Verification items for the finished model (mm, model axes). Face numbers are marked on the shaded views. A direction names the side the tool comes from. Give positions to 0.01 mm unless a question says otherwise; leave off trailing zeros. Order: outer loops, then holes, each group sorted by start corner. A loop starts at its lowest first (then second) coordinate and runs counter-clockwise, first axis right, second up. Notation, with made-up numbers: (81.5, -8.5) -> (86.5, -8.5) arc R28 cw to (86.5, 14.5) -> close; hole circle Ø9 at (7, -24). An arc over 180 degrees is marked (long way). Return JSON: item names as keys, results as strings. Group by question number.
(1) Tool access check on the marked faces 1 and 2. Record the directions out of +Z, -Z, +X, -X, +Y, -Y that give a thin tool (end or side, any length) a straight path to the whole face; none if there is none.
(2) Cross-section at A-A on y = 0. Enter the section's corners in (x, z).
(3) Thickness scan on line 1 along Z through (x, y) = (9.75, 0.25); line 2 along Y through (x, z) = (1.25, 3.5); line 3 along Y through (x, z) = (4.75, 4.75). Record the ranges inside material, lowest first.
(4) Depth check by flat-ended pin: pin 1 Ø3 at (x, z) = (4.5, 9) entering from +Y; pin 2 Ø1 at (y, z) = (7.5, 13) entering from +X; pin 3 Ø1.5 at (y, z) = (10, 9) entering from +X. Enter the tip coordinate at first touch or a pass-through.
(5) Cross-section at B-B on z = 13.5. Enter the section's corners in (x, y).
(6) Release check for a two-part mould opening along Y. For the marked faces 3, 4 and 5 record: pulls with the +Y half, pulls with the -Y half, needs draft (parallel to the pull), parting line crosses it, or undercut.
Autodesk Fusion 360 part; units mm, degrees
sketch "Sketch1" plane through (0, 0, 0) normal (1, 0, 0) x (0, 1, 0)
  line L0 (0, 0) -> (-26.3359, 0) construction
  line L1 (-11.25, 0) -> (-11.25, 17.5)
  line L2 (-11.25, 17.5) -> (-6.25, 17.5)
  line L3 (-11.25, 0) -> (-14.25, 0)
  line L4 (-14.25, 0) -> (-14.25, 20.5)
  line L5 (-14.25, 20.5) -> (-6.25, 20.5)
  line L6 (-6.25, 20.5) -> (-6.25, 17.5)
  line L7 (0, 0) -> (0, 80.4746)
  dimension "d1" = 17.5
  dimension "d3" = 22.5
  dimension "d4" = 12.5
  dimension "d5" = 3
  dimension "d6" = 3
revolve "Revolve1" add sketch "Sketch1" angle 180 about axis through (0, 0, 0) along (0, 0, 1)
chamfer "Chamfer1" distance 1 distance2 2 1 edges at (14.25, 0, 20.5) measured on face at (2.7221, 11.2267, 20.5)
chamfer "Chamfer2" distance 1 distance2 1 1 edges at (11.25, 0, 17.5) measured on face at (6.7928, 8.9677, 5.8333)
equation "d6 = d5"
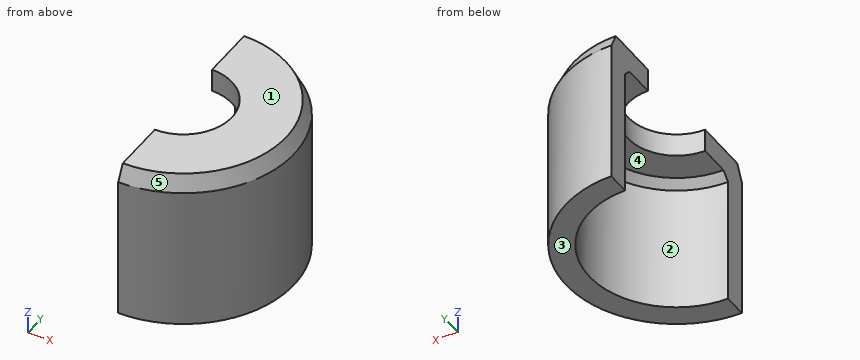
Verdict:
{
 "1": {"face 1": "+Z, +X, -X, +Y, -Y", "face 2": "-Z, -X"},
 "2": {"outline": "(6.25, 17.5) -> (10.25, 17.5) -> (11.25, 16.5) -> (11.25, 0) -> (14.25, 0) -> (14.25, 18.5) -> (13.25, 20.5) -> (6.25, 20.5) -> close"},
 "3": {"line 1": "17.5 to 20.5", "line 2": "-14.2 to -11.18, 11.18 to 14.2", "line 3": "-13.44 to -10.2, 10.2 to 13.44"},
 "4": {"pin 1": "y = 13.93", "pin 2": "x = 12.41", "pin 3": "x = 10.84"},
 "5": {"outline": "(0, -14.25) arc R14.25 ccw to (0, 14.25) -> (0, 11.25) arc R11.25 cw to (0, -11.25) -> close"},
 "6": {"face 3": "needs draft", "face 4": "undercut", "face 5": "parting line crosses it"}
}
